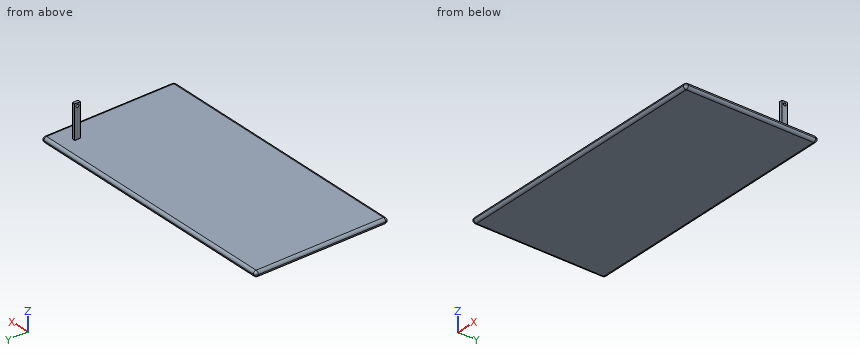
Autodesk Inventor part; units mm, degrees
ref_plane "YZ Plane" through (0, 0, 0) normal (1, 0, 0) x (0, 1, 0)
ref_plane "XZ Plane" through (0, 0, 0) normal (0, 1, 0) x (-1, 0, 0)
ref_plane "XY Plane" through (0, 0, 0) normal (0, 0, 1) x (1, 0, 0)
sketch "Sketch1" plane through (0, 0, 0) normal (0, 0, 1) x (1, 0, 0)
  line L0 (0, 0) -> (1219.2, 0)
  line L1 (1219.2, 0) -> (1219.2, 609.6)
  line L2 (1219.2, 609.6) -> (0, 609.6)
  line L3 (0, 609.6) -> (0, 0)
  dimension "d0" = 1219.2
  dimension "d1" = 609.6
extrude "Extrusion1" add sketch "Sketch1" along normal blind 25.4
fillet "Fillet1" radius 12.7 12 edges at (609.6, 609.6, 25.4) (609.6, 609.6, 0) (1219.2, 304.8, 25.4) (1219.2, 304.8, 0) (1219.2, 609.6, 12.7) (0, 609.6, 12.7) (0, 304.8, 25.4) (0, 304.8, 0) (609.6, 0, 0) (609.6, 0, 25.4) (0, 0, 12.7) (1219.2, 0, 12.7)
sketch "Sketch3" plane through (0, 0, 25.4) normal (0, 0, 1) x (1, 0, 0)
  line L0 (1134.1424, 536.1398) -> (1121.4424, 536.1398)
  line L1 (1121.4424, 536.1398) -> (1121.4424, 510.7398)
  line L2 (1121.4424, 510.7398) -> (1134.1424, 510.7398)
  line L3 (1134.1424, 510.7398) -> (1134.1424, 536.1398)
  point P0 (0, 0)
  dimension "d11" = 12.7
  dimension "d12" = 25.4
extrude "Extrusion3" add sketch "Sketch3" along normal blind 152.4
sketch "Sketch4" plane through (1121.4424, 510.7398, 25.4) normal (-1, 0, 0) x (0, 0, 1)
  circle A0 centre (139.7, 12.7) radius 6.35
  line L0 (0, 25.4) -> (152.4, 25.4)
  line L1 (0, 0) -> (152.4, 0)
  line L2 (152.4, 25.4) -> (152.4, 0)
  point P0 (-25.4, -510.7398)
  dimension "d15" = 12.7
  dimension "d16" = 25.4
  dimension "d17" = 12.7
  dimension "d18" = 12.7
extrude "Extrusion4" cut sketch "Sketch4" against normal through all
properties part number "BasePlate"
Work out the finished part from the listing and answer in its coordinate system (mm). Coordinates: 2 decimals unless noted, no trailing zeros. Loops run counter-clockwise (first coordinate to the right, second up) from the corner with the lowest first, then second, coordinate; pieces in that order, holes last. Notation, with made-up numbers: M -13,39.25 L -5,39.25 A14 cw -5,50.25 Z; hole C -3.5,-30.75 d9. An arc over 180 degrees is marked long. Use CSV: the item, a comma, the result in double quotes. Start each with the question number.
(1) Consider line 1 (Y direction, x = 1127.5, z = 165.1); line 2 (Z direction, x = 822, y = 518.5); line 3 (Y direction, x = 1155, z = 18). Determine where each line is inside the solid, lowest interval first.
(2) Find section C-C, the plane z = 94.5. Give the vertices of the cut face in (x, y).
(3) Given pin 1 Ø20.5 at (y, z) = (520.5, 131) entering from -X; pin 2 Ø14 at (x, z) = (1130, 106.5) entering from +Y; pin 3 Ø14 at (x, z) = (1127, 122) entering from -Y; pin 4 Ø1.5 at (x, y) = (439, 451) entering from -Z, each flat-ended and moving along its own axis, determine where each tip first touches the part or whether it passes through.
Recorded:
1,line 1,"y = 510.74 to 517.09, 529.79 to 536.14"
1,line 2,"z = 0 to 25.4"
1,line 3,"y = 1.16 to 608.44"
2,outline,"M 1121.44,510.74 L 1134.14,510.74 L 1134.14,536.14 L 1121.44,536.14 Z"
3,pin 1,"stops at x = 1121.44"
3,pin 2,"stops at y = 536.14"
3,pin 3,"stops at y = 510.74"
3,pin 4,"stops at z = 0"
